Check sheet for the modelled part. Datum: model origin and axes. Units: mm. Face numbers are marked on the shaded views. A direction names the side the tool comes from. Give positions to 0.01 mm unless a question says otherwise; leave off trailing zeros. Write each loop counter-clockwise with the first axis right and the second up, starting at its lowest first coordinate (ties: lowest second). Pieces come first, ordered by that corner, then holes. Notation, with made-up numbers: (36, 64) - (65, 64) arc R17 ccw to (65, 68) - close; hole circle Ø11 at (21.25, 56.25). An arc over 180 degrees is marked (long way). Return JSON: item names as keys, results as strings. Group by question number.
```python
from build123d import *

# Parameters (mm, degrees)
SKETCH1_W           = 9
SKETCH1_H           = 8.8
BOSS_EXTRUDE1_DEPTH = 6
SKETCH2_W           = 1
SKETCH2_H           = 3.86
CUT_EXTRUDE1_DEPTH  = 12.562439189
LPATTERN1_COUNT     = 4
LPATTERN1_PITCH     = 2
FILLET1_R           = 0.25
FILLET2_R           = 0.5


with BuildPart() as part:
    # Sketch1 → Boss-Extrude1 (new body)
    with BuildSketch(Plane(origin=(0, 0, 0), x_dir=(1, 0, 0), z_dir=(0, 1, 0))):
        Rectangle(SKETCH1_W, SKETCH1_H)
    extrude(amount=BOSS_EXTRUDE1_DEPTH)

    # Sketch2 → Cut-Extrude1 (cut, through all)
    with BuildSketch(Plane.XY.offset(4.4)):
        with Locations((-3, 4.07)):
            Rectangle(SKETCH2_W, SKETCH2_H)
    cut_extrude1 = extrude(amount=-CUT_EXTRUDE1_DEPTH, mode=Mode.SUBTRACT)

    # LPattern1: Cut-Extrude1 ×4
    with Locations(*[(i * LPATTERN1_PITCH, 0, 0) for i in range(1, LPATTERN1_COUNT)]):
        add(cut_extrude1, mode=Mode.SUBTRACT)

    # Fillet1
    fillet1_edges = [part.edges().sort_by_distance(p)[0] for p in [
        (-2.5, 2.14, 0),
        (-3.5, 2.14, 0),
        (-0.5, 2.14, 0),
        (-1.5, 2.14, 0),
        (1.5, 2.14, 0),
        (0.5, 2.14, 0),
        (3.5, 2.14, 0),
        (2.5, 2.14, 0),
    ]]
    fillet(fillet1_edges, radius=FILLET1_R)

    # Fillet2
    fillet2_edges = [part.edges().sort_by_distance(p)[0] for p in [
        (-4.5, 6, 0),
        (-3.5, 6, 0),
        (-2.5, 6, 0),
        (-1.5, 6, 0),
        (-0.5, 6, 0),
        (0.5, 6, 0),
        (1.5, 6, 0),
        (2.5, 6, 0),
        (3.5, 6, 0),
        (4.5, 6, 0),
        (-4.5, 0, 0),
        (4.5, 0, 0),
    ]]
    fillet(fillet2_edges, radius=FILLET2_R - 0.0001)  # a hair under: the kernel refuses the full size


solid = part.part
```
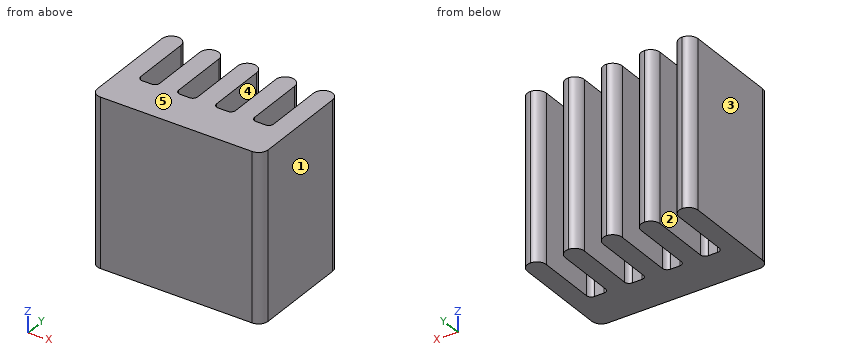
Item 1: Section check B-B on x = 1. Record the cut outline in (y, z).
Item 2: Mould release check, pull along X, two halves, no side actions. Record for the marked faces 3, 4 and 5: +X half, -X half, draft (parallel to the pull), parting line (faces both ways), or undercut.
Item 3: Depth check by flat-ended pin: pin 1 (0.6 mm diameter, centred on x = 3, z = -1.5, fed in from +Y). Enter the tip coordinate at first touch or a pass-through.
Item 4: Section check A-A on y = 5.2. Record the cut outline in (x, z).
Item 5: Access from +Z, -Z, +X, -X, +Y, -Y to the whole of each face (thin tool, end or side, straight path). Record for the marked faces 1 and 2.
Item 6: Material ranges on line 1 along X through (y, z) = (4.85, 3.25); line 2 along X through (y, z) = (0.45, -2); line 3 along Y through (x, z) = (3.25, -3), recorded low to high. Write a range as from..to.
Reply:
{
 "1": {"outline": "(0, -4.4) - (2.14, -4.4) - (2.14, 4.4) - (0, 4.4) - close"},
 "2": {"face 3": "-X half", "face 4": "undercut", "face 5": "draft"},
 "3": {"pin 1": "y = 2.15"},
 "4": {"outline": "(-4.5, -4.4) - (-3.5, -4.4) - (-3.5, 4.4) - (-4.5, 4.4) - close; (-2.5, -4.4) - (-1.5, -4.4) - (-1.5, 4.4) - (-2.5, 4.4) - close; (-0.5, -4.4) - (0.5, -4.4) - (0.5, 4.4) - (-0.5, 4.4) - close; (1.5, -4.4) - (2.5, -4.4) - (2.5, 4.4) - (1.5, 4.4) - close; (3.5, -4.4) - (4.5, -4.4) - (4.5, 4.4) - (3.5, 4.4) - close"},
 "5": {"face 1": "+Z, -Z, +X, +Y, -Y", "face 2": "+Z, -Z, +Y"},
 "6": {"line 1": "-4.5..-3.5, -2.5..-1.5, -0.5..0.5, 1.5..2.5, 3.5..4.5", "line 2": "-4.5..4.5", "line 3": "0..2.14"}
}
